Input: dimensioned drawing with shaded views. Units: mm. Origin: part minimum x, y, z. Round coordinates to 2 decimals unless told otherwise and drop trailing zeros. Loops run counter-clockwise (first coordinate to the right, second up) from the corner with the lowest first, then second, coordinate; pieces in that order, holes last. Notation, with made-up numbers: M -40,39 L -23,39 A21 ccw -23,66 Z; hole C 24.5,-7 d10. An arc over 180 degrees is marked long. Use one line per item in the form item = value. Start each with the question number.
Q1. Section query A-A, the plane x = 38.1. Output: boundary loops of the cut face in (y, z) (1 decimal), and give its area (3 significant figures).
Q2. Section query D-D, the plane y = 18. Output: boundary loops of the cut face in (x, z) (1 decimal).
Q3. Section query C-C, the plane x = 19. Output: boundary loops of the cut face in (y, z) (1 decimal), and give its area (3 significant figures).
Q4. First-contact query: P1, Ø1, axis at x = 51, z = 1, coming from the +Y side (1 decimal); P2, Ø1, axis at y = 45, z = 2, coming from the +X side; P3, Ø1.6, axis at x = 36.5, z = 1, coming from the +Y side. Flat tips, straight axial feed; report the tip coordinate or a pass-through.
Q5. Ray query, line 1 along Y through (x, z) = (30.5, 1) (1 decimal); line 2 along Y through (x, z) = (46.5, 1.15) (1 decimal); line 3 along Y through (x, z) = (38.5, 0.7). Return the intervals inside material, ascending.
Q6. Section query B-B, the plane z = 2.25. State how many separate pieces and enclosed holes the cut face has, and give its area (3 significant figures).
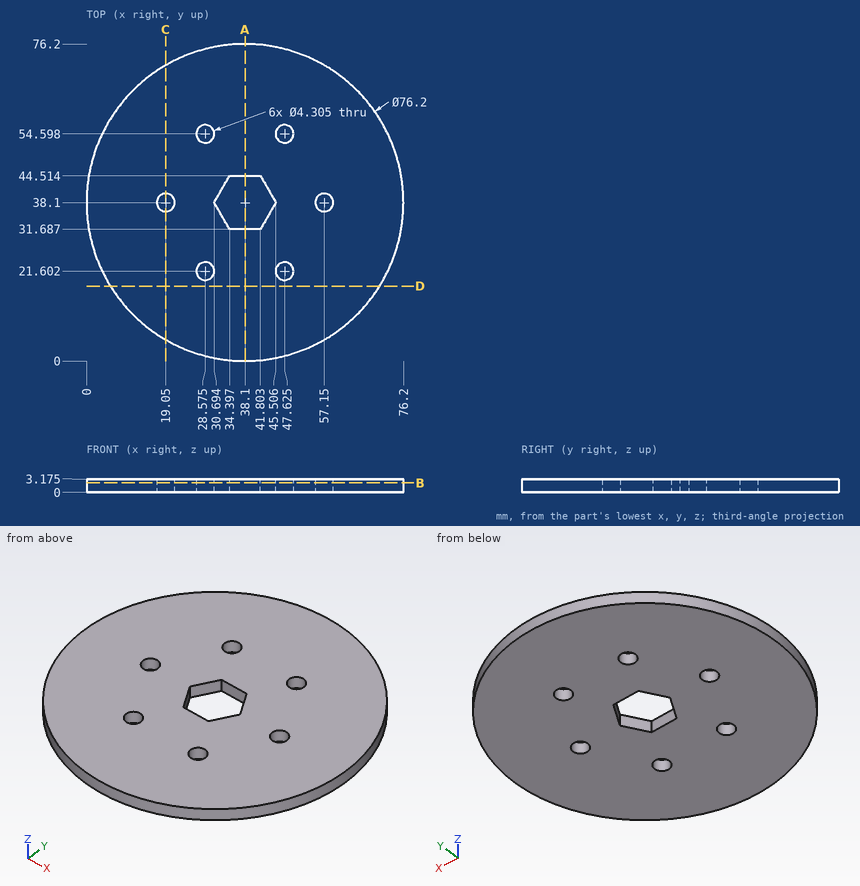
Results found:
q1.outline = M 0,0 L 31.7,0 L 31.7,3.2 L 0,3.2 Z; M 44.5,0 L 76.2,0 L 76.2,3.2 L 44.5,3.2 Z
q1.area = 201 mm²
q2.outline = M 5.7,0 L 70.5,0 L 70.5,3.2 L 5.7,3.2 Z
q3.outline = M 5.1,0 L 35.9,0 L 35.9,3.2 L 5.1,3.2 Z; M 40.3,0 L 71.1,0 L 71.1,3.2 L 40.3,3.2 Z
q3.area = 196 mm²
q4.P1 = 74.1
q4.P2 = 75.66
q4.P3 = 76.19
q5.line_1 = 0.8 to 20.6, 22.6 to 53.6, 55.6 to 75.4
q5.line_2 = 0.9 to 19.8, 23.4 to 52.8, 56.4 to 75.3
q5.line_3 = 0 to 31.69, 44.51 to 76.2
q6.separate_pieces = 1
q6.enclosed_holes = 7
q6.area = 4,330 mm²
